Work out the finished part from the listing and answer in its coordinate system (mm). Face numbers are marked on the shaded views. A direction names the side the tool comes from. Round coordinates to 2 decimals unless told otherwise and drop trailing zeros. Write each loop counter-clockwise with the first axis right and the second up, starting at its lowest first coordinate (ties: lowest second). Pieces come first, ordered by that corner, then holes.
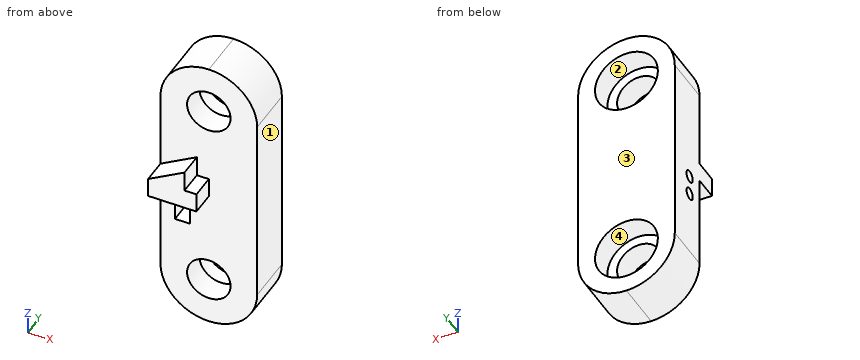
from build123d import *

# Parameters (mm, degrees)
SKETCH_1_W          = 20
SKETCH_1_H          = 10
EXTRUDE_1_DEPTH     = 59.939609738
SKETCH_2_R          = 6.5
CUT_EXTRUDE_1_DEPTH = 5
SKETCH_3_R          = 4.5
CUT_EXTRUDE_2_DEPTH = 20
CUT_EXTRUDE_3_DEPTH = 10
EXTRUDE_2_DEPTH     = 5
SKETCH_5_W          = 3.108428341
SKETCH_5_H          = 8
CUT_EXTRUDE_4_DEPTH = 8
SKETCH_7_R          = 1.25
CUT_EXTRUDE_5_DEPTH = 8


with BuildPart() as part:
    # Sketch 1 → Extrude 1 (new body)
    with BuildSketch(Plane.XY):
        Rectangle(SKETCH_1_W, SKETCH_1_H)
    extrude(amount=EXTRUDE_1_DEPTH)

    # Sketch 2 → Cut-Extrude 1 (cut)
    with BuildSketch(Plane(origin=(0, 5, 0), x_dir=(1, 0, 0), z_dir=(0, 1, 0))):
        with Locations(Location((0, -10, 0), (0, 0, 270))):
            Circle(SKETCH_2_R)
    cut_extrude_1 = extrude(amount=-CUT_EXTRUDE_1_DEPTH, mode=Mode.SUBTRACT)

    # Sketch 3 → Cut-Extrude 2 (cut)
    with BuildSketch(Plane(origin=(0, 5, 0), x_dir=(1, 0, 0), z_dir=(0, 1, 0))):
        with Locations(Location((0, -10, 0), (0, 0, 270))):
            Circle(SKETCH_3_R)
    cut_extrude_2 = extrude(amount=-CUT_EXTRUDE_2_DEPTH, mode=Mode.SUBTRACT)

    # Sketch 3_4 → Cut-Extrude 3 (cut)
    with BuildSketch(Plane(origin=(0, 5, 0), x_dir=(1, 0, 0), z_dir=(0, 1, 0))):
        with BuildLine():
            Line((-10, 0), (-10, -10))
            ThreePointArc((-10, -10), (-7.071067806, -2.928932182), (1.6e-08, 0))
            Line((1.6e-08, 0), (-10, 0))
        make_face()
        with BuildLine():
            Line((10, 0), (1.6e-08, 0))
            ThreePointArc((1.6e-08, 0), (7.071067818, -2.928932194), (10, -10))
            Line((10, -10), (10, 0))
        make_face()
    cut_extrude_3 = extrude(amount=-CUT_EXTRUDE_3_DEPTH, mode=Mode.SUBTRACT)

    # Mirror 1: Cut-Extrude 1, Cut-Extrude 2, Cut-Extrude 3 across plane
    add(cut_extrude_1.mirror(Plane.XY.offset(29.969804869)), mode=Mode.SUBTRACT)
    add(cut_extrude_2.mirror(Plane.XY.offset(29.969804869)), mode=Mode.SUBTRACT)
    add(cut_extrude_3.mirror(Plane.XY.offset(29.969804869)), mode=Mode.SUBTRACT)

    # Sketch 4 → Extrude 2 (add)
    with BuildSketch(Plane(origin=(0, -5, 0), x_dir=(1, 0, 0), z_dir=(0, 1, 0))):
        Polygon((-2.475489913, -38.118080125), (-10, -33.773802201), (-10, -29.747626971), (0, -29.747626971), (0, -33.840387137), (-2.475489913, -33.840387137), align=None)
    extrude(amount=-EXTRUDE_2_DEPTH)

    # Sketch 5 → Cut-Extrude 4 (cut)
    with BuildSketch(Plane.XZ.offset(5)):
        with Locations((-5.44578583, 25.747626971)):
            Rectangle(SKETCH_5_W, SKETCH_5_H)
    extrude(amount=-CUT_EXTRUDE_4_DEPTH, mode=Mode.SUBTRACT)

    # Sketch 7 → Cut-Extrude 5 (cut)
    with BuildSketch(Plane(origin=(-7, 0, 0), x_dir=(0, 0, -1), z_dir=(1, 0, 0))):
        with Locations((-23.689322855, -1)):
            Circle(SKETCH_7_R)
        with Locations((-27.805931086, -1)):
            Circle(SKETCH_7_R)
    extrude(amount=-CUT_EXTRUDE_5_DEPTH, mode=Mode.SUBTRACT)


solid = part.part
Q1. A tool of negligible diameter and unlimited length cuts with its end or side. For the marked faces 3 and 4, from which of +Z, -Z, +X, -X, +Y, -Y can it reach the whole face along a straight path? Write none if from no direction.
Q2. Find the intervals of material crossed by L1, parallel to X at y = -2.3, z = 10; L2, parallel to Y at x = -6.5, z = 12.5; L3, parallel to X at y = -3.25, z = 52, in increasing order.
Q3. Find section C-C (z = 26). Determine the outline of the cut face in (x, y).
Q4. Find section B-B (y = 2). Determine the outline of the cut face in (x, z), plus the area to 3 significant figures.
Q5. The mould has two halves that part along Z. Classify the marked faces 1 and 2: +Z half, -Z half, draft (parallel to the pull), parting line (faces both ways), or undercut.
Q6. Find section A-A (y = -1). Determine the outline of the cut face in (x, z).
Q7. Find section D-D (x = -8.5). Determine the outline of the cut face in (y, z), plus the area to 3 significant figures.
Q8. Given pin 1 (4 mm diameter, centred on x = -3, y = -5.5, fed in from +Z); pin 2 (10.5 mm diameter, centred on x = 0, z = 49.94, fed in from +Y); pin 3 (2.5 mm diameter, centred on x = -5.5, y = 0.5, fed in from +Z), each flat-ended and moving along its own axis, determine where each tip first touches the part or whether it passes through.
Report:
1. face 3: +Z, -Z, +X, -X, +Y
1. face 4: +Y
2. L1: x = -10 to -4.5, 4.5 to 10
2. L2: y = -5 to 5
2. L3: x = -9.79 to -4, 4 to 9.79
3. outline: (-10, -5) - (-7, -5) - (-7, 3) - (-3.89, 3) - (-3.89, -5) - (10, -5) - (10, 5) - (-10, 5) - close
4. outline: (-10, 10) arc R10 ccw to (10, 10) - (10, 49.94) arc R10 ccw to (-10, 49.94) - close; hole (-7, 21.75) - (-3.89, 21.75) - (-3.89, 29.75) - (-7, 29.75) - close; hole circle Ø13 at (0, 10); hole circle Ø13 at (0, 49.94)
4. area: 823 mm2
5. face 1: draft
5. face 2: undercut
6. outline: (-10, 10) arc R10 ccw to (10, 10) - (10, 49.94) arc R10 ccw to (-10, 49.94) - (-10, 29.06) - (-7, 29.06) - (-7, 29.75) - (-3.89, 29.75) - (-3.89, 21.75) - (-7, 21.75) - (-7, 22.44) - (-10, 22.44) - close; (-10, 24.94) - (-7, 24.94) - (-7, 26.56) - (-10, 26.56) - close; hole circle Ø9 at (0, 10); hole circle Ø9 at (0, 49.94)
7. outline: (-10, 29.75) - (-5, 29.75) - (-5, 4.73) - (5, 4.73) - (5, 55.21) - (-5, 55.21) - (-5, 34.64) - (-10, 34.64) - close; hole circle Ø2.5 at (-1, 23.69); hole circle Ø2.5 at (-1, 27.81)
7. area: 519 mm2
8. pin 1: stops at z = 59.88
8. pin 2: stops at y = 0
8. pin 3: stops at z = 58.99
